Input: part model. Units: mm. Frame: model coordinates. Face numbers are marked on the shaded views. A direction names the side the tool comes from. Coordinates: 2 decimals unless noted, no trailing zeros. Order: outer loops, then holes, each group sorted by start corner. A loop starts at its lowest first (then second) coordinate and runs counter-clockwise, first axis right, second up. Notation, with made-up numbers: M -17.75,-15 L -12.75,-15 A13 cw -12.75,6 Z; hole C -25.5,11.5 d5. An arc over 180 degrees is marked long. One line per item, written item: value.
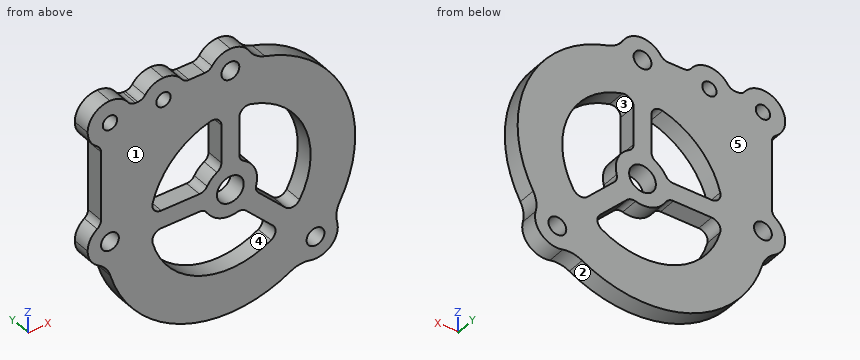
```python
from build123d import *

# Parameters (mm, degrees)
BOSS_EXTRUDE1_DEPTH         = 6.35
SKETCH2_R                   = 4.7625
CUT_EXTRUDE1_DEPTH          = 7.35
F_1_4_0_25_DIAMETER_HOLE1_D = 6.35
CUT_EXTRUDE2_DEPTH          = 7.35
FILLET1_R                   = 3.175
BOSS_EXTRUDE2_DEPTH         = 6.35
F_10_CLEARANCE_HOLE1_D      = 5.1054
CUT_EXTRUDE5_DEPTH          = 6.35
FILLET3_R                   = 3.175


with BuildPart() as part:
    # Sketch1 → Boss-Extrude1 (new body)
    with BuildSketch(Plane(origin=(0, 0, 0), x_dir=(1, 0, 0), z_dir=(0, 1, 0))):
        with BuildLine():
            ThreePointArc((-42.706862745, -12.325841735), (-31.430896424, -31.430896424), (-12.325841735, -42.706862745))
            ThreePointArc((-12.325841735, -42.706862745), (-9.162618669, -44.306267621), (-6.803224334, -46.951515152))
            ThreePointArc((-6.803224334, -46.951515152), (0, -50.8), (6.803224334, -46.951515152))
            ThreePointArc((6.803224334, -46.951515152), (9.162618669, -44.306267621), (12.325841735, -42.706862745))
            ThreePointArc((12.325841735, -42.706862745), (41.06644522, -17.010278569), (38.913998525, 21.482625976))
            ThreePointArc((38.913998525, 21.482625976), (37.808212078, 24.85031249), (38.010340811, 28.38912869))
            ThreePointArc((38.010340811, 28.38912869), (35.921024484, 35.921024484), (28.38912869, 38.010340811))
            ThreePointArc((28.38912869, 38.010340811), (24.85031249, 37.808212078), (21.482625976, 38.913998525))
            ThreePointArc((21.482625976, 38.913998525), (-17.010278569, 41.06644522), (-42.706862745, 12.325841735))
            ThreePointArc((-42.706862745, 12.325841735), (-44.306267621, 9.162618669), (-46.951515152, 6.803224334))
            ThreePointArc((-46.951515152, 6.803224334), (-50.8, 0), (-46.951515152, -6.803224334))
            ThreePointArc((-46.951515152, -6.803224334), (-44.306267621, -9.162618669), (-42.706862745, -12.325841735))
        make_face()
    extrude(amount=BOSS_EXTRUDE1_DEPTH)

    # Sketch2 → Cut-Extrude1 (cut, through all)
    with BuildSketch(Plane(origin=(0, 6.35, 0), x_dir=(1, 0, 0), z_dir=(0, 1, 0))):
        Circle(SKETCH2_R)
    extrude(amount=-CUT_EXTRUDE1_DEPTH, mode=Mode.SUBTRACT)

    # 1/4 (0.25) Diameter Hole1 (through all)
    with Locations(Plane(origin=(0, 6.35, 0), x_dir=(1, 0, 0), z_dir=(0, 1, 0))):
        with Locations((-42.8625, 0), (30.308364409, 30.308364409), (0, -42.8625)):
            Hole(F_1_4_0_25_DIAMETER_HOLE1_D / 2)

    # Sketch5 → Cut-Extrude2 (cut, through all)
    with BuildSketch(Plane(origin=(0, 6.35, 0), x_dir=(1, 0, 0), z_dir=(0, 1, 0))):
        with BuildLine():
            Line((-28.398063314, 3.175), (-8.980256121, 3.175))
            ThreePointArc((-8.980256121, 3.175), (-3.645059693, 8.799952547), (4.10493597, 8.59506403))
            Line((4.10493597, 8.59506403), (17.835399112, 22.325527172))
            ThreePointArc((17.835399112, 22.325527172), (-10.93517908, 26.399857642), (-28.398063314, 3.175))
        make_face()
        with BuildLine():
            Line((-28.398063314, -3.175), (-8.980256121, -3.175))
            ThreePointArc((-8.980256121, -3.175), (-6.735192091, -6.735192091), (-3.175, -8.980256121))
            Line((-3.175, -8.980256121), (-3.175, -28.398063314))
            ThreePointArc((-3.175, -28.398063314), (-20.205576272, -20.205576272), (-28.398063314, -3.175))
        make_face()
        with BuildLine():
            Line((22.325527172, 17.835399112), (8.59506403, 4.10493597))
            ThreePointArc((8.59506403, 4.10493597), (8.799952547, -3.645059693), (3.175, -8.980256121))
            Line((3.175, -8.980256121), (3.175, -28.398063314))
            ThreePointArc((3.175, -28.398063314), (26.399857642, -10.93517908), (22.325527172, 17.835399112))
        make_face()
    extrude(amount=-CUT_EXTRUDE2_DEPTH, mode=Mode.SUBTRACT)

    # Fillet1
    fillet1_edges = [part.edges().sort_by_distance(p)[0] for p in [
        (22.325527172, 3.175, -17.835399112),
        (3.175, 3.175, 28.398063314),
        (3.175, 3.175, 8.980256121),
        (8.59506403, 3.175, -4.10493597),
        (-3.175, 3.175, 28.398063314),
        (-28.398063314, 3.175, 3.175),
        (-8.980256121, 3.175, 3.175),
        (-3.175, 3.175, 8.980256121),
        (-28.398063314, 3.175, -3.175),
        (17.835399112, 3.175, -22.325527172),
        (4.10493597, 3.175, -8.59506403),
        (-8.980256121, 3.175, -3.175),
    ]]
    fillet(fillet1_edges, radius=FILLET1_R)

    # Sketch8 → Boss-Extrude2 (add)
    with BuildSketch(Plane(origin=(0, 6.35, 0), x_dir=(1, 0, 0), z_dir=(0, 1, 0))):
        with BuildLine():
            Line((-50.8, 0), (-50.8, -42.8625))
            ThreePointArc((-50.8, -42.8625), (-48.475160076, -48.475160076), (-42.8625, -50.8))
            Line((-42.8625, -50.8), (0, -50.8))
            ThreePointArc((0, -50.8), (-3.908154839, -49.771206971), (-6.803224334, -46.951515152))
            ThreePointArc((-6.803224334, -46.951515152), (-9.162618669, -44.306267621), (-12.325841735, -42.706862745))
            ThreePointArc((-12.325841735, -42.706862745), (-31.430896424, -31.430896424), (-42.706862745, -12.325841735))
            ThreePointArc((-42.706862745, -12.325841735), (-44.306267621, -9.162618669), (-46.951515152, -6.803224334))
            ThreePointArc((-46.951515152, -6.803224334), (-49.771206971, -3.908154839), (-50.8, 0))
        make_face()
    extrude(amount=-BOSS_EXTRUDE2_DEPTH)

    # #10 Clearance Hole1 (through all)
    with Locations(Plane(origin=(0, 6.35, 0), x_dir=(1, 0, 0), z_dir=(0, 1, 0))):
        with Locations((-42.8625, -42.8625), (-23.8125, -42.8625)):
            Hole(F_10_CLEARANCE_HOLE1_D / 2)

    # Sketch15 → Cut-Extrude5 (cut)
    with BuildSketch(Plane(origin=(0, 6.35, 0), x_dir=(1, 0, 0), z_dir=(0, 1, 0))):
        with BuildLine():
            ThreePointArc((-46.0375, -35.587661084), (-49.503488961, -38.5149522), (-50.8, -42.8625))
            Line((-50.8, -42.8625), (-50.8, 0))
            ThreePointArc((-50.8, 0), (-49.503488961, -4.3475478), (-46.0375, -7.274838916))
            Line((-46.0375, -7.274838916), (-46.0375, -35.587661084))
        make_face()
        with BuildLine():
            Line((-31.087338916, -46.0375), (-35.587661084, -46.0375))
            ThreePointArc((-35.587661084, -46.0375), (-38.5149522, -49.503488961), (-42.8625, -50.8))
            Line((-42.8625, -50.8), (-23.8125, -50.8))
            ThreePointArc((-23.8125, -50.8), (-28.1600478, -49.503488961), (-31.087338916, -46.0375))
        make_face()
        with BuildLine():
            ThreePointArc((-16.537661084, -46.0375), (-19.4649522, -49.503488961), (-23.8125, -50.8))
            Line((-23.8125, -50.8), (0, -50.8))
            ThreePointArc((0, -50.8), (-4.3475478, -49.503488961), (-7.274838916, -46.0375))
            Line((-7.274838916, -46.0375), (-16.537661084, -46.0375))
        make_face()
    extrude(amount=-CUT_EXTRUDE5_DEPTH, mode=Mode.SUBTRACT)

    # Fillet3
    fillet3_edges = [part.edges().sort_by_distance(p)[0] for p in [
        (-46.0375, 3.175, 35.587661084),
        (-46.0375, 3.175, 7.274838916),
        (-35.587661084, 3.175, 46.0375),
        (-31.087338916, 3.175, 46.0375),
        (-16.537661084, 3.175, 46.0375),
        (-7.274838916, 3.175, 46.0375),
    ]]
    fillet(fillet3_edges, radius=FILLET3_R)


solid = part.part
```
(1) Cut plane B-B on y = 4. Give the number of separate pieces and of enclosed holes in the cut face, plus the area to 3 significant figures.
Data:
separate pieces: 1
enclosed holes: 9
area: 5,040 mm2
(2) First-contact query: pin 1 (3 mm diameter, centred on y = 2.5, z = -23, fed in from -X); pin 2 (1.7 mm diameter, centred on x = -10.5, y = 2, fed in from +Z); pin 3 (3 mm diameter, centred on y = 2.5, z = 15, fed in from -X). Flat tips, straight axial feed; report the tip coordinate or a pass-through.
Data:
pin 1: stops at x = -38.9
pin 2: stops at z = 46.04
pin 3: stops at x = -46.04
(3) Draft query along Z for the marked faces 1, 2 and 3. Return one class per face: released by +Z, released by -Z, zero draft, split by the parting line, or undercut.
Data:
face 1: zero draft
face 2: released by -Z
face 3: undercut
(4) Access query for the marked faces 4 and 5. Directions: +Z, -Z, +X, -X, +Y, -Y. A direction counts if a zero-diameter tool reaches every point of the face in a straight line with its end or side. Return the directions, or none.
Data:
face 4: +Y, -Y
face 5: +Z, -Z, +X, -X, +Y
(5) Cut plane A-A on x = 30. Output: boundary loops of the cut face in (y, z).
Data:
outline: M 0,-38.24 L 6.35,-38.24 L 6.35,-33.47 L 0,-33.47 Z; M 0,-27.15 L 6.35,-27.15 L 6.35,32.8 L 0,32.8 Z
(6) Ray query, line 1 (Z direction, x = -16, y = 1) (1 decimal); line 2 (X direction, y = 4.5, z = 25.5); line 3 (Z direction, x = 15, y = 3.75). Return the intervals inside material, ascending. Write a range as from..to.
Data:
line 1: z = -41.5..-23.7, -3.2..3.2, 23.7..46.3
line 2: x = -46.04..-12.89, -3.31..3.31, 12.89..36.41
line 3: z = -41.84..-24.26, -19.49..-10.51, 24.32..41.84
